from build123d import *

# Parameters (mm, degrees)
F0_R     = 2.54
F1_DEPTH = 2.54
F2_R     = 10.16
F3_DEPTH = 1.27


# Not quite as in the source:
# - a feature names something its author has since deleted; it is built from what else it names


with BuildPart() as f1:
    # F0 (on Front) → F1 (new body)
    with BuildSketch(Plane.XZ):
        with BuildLine():
            ThreePointArc((23.9710795428, 0.5081666473), (11.7817898671, 6.8022195513), (12.4256249974, 20.5054805165))
            ThreePointArc((12.4256249974, 20.5054805165), (0, 44.5693936748), (-12.4256249974, 20.5054805165))
            ThreePointArc((-12.4256249974, 20.5054805165), (-11.7817898671, 6.8022195513), (-23.9710795428, 0.5081666473))
            ThreePointArc((-23.9710795428, 0.5081666473), (-38.5982271537, -22.2846968374), (-11.5454545455, -21.0136471639))
            ThreePointArc((-11.5454545455, -21.0136471639), (0, -13.6044391026), (11.5454545455, -21.0136471639))
            ThreePointArc((11.5454545455, -21.0136471639), (38.5982271537, -22.2846968374), (23.9710795428, 0.5081666473))
        make_face()
        Circle(F0_R, mode=Mode.SUBTRACT)
    extrude(amount=F1_DEPTH)

    # F2 (on face) → F3 (cut)
    with BuildSketch(Plane(origin=(0, 0, 0), x_dir=(-1, 0, 0), z_dir=(0, 1, 0))):
        with Locations((25.4, -14.6646968374)):
            Circle(F2_R)
        with Locations((0, 29.3293936748)):
            Circle(F2_R)
        with Locations((-25.4, -14.6646968374)):
            Circle(F2_R)
    extrude(amount=-F3_DEPTH, mode=Mode.SUBTRACT)


solid = f1.part
CAD build for the part. Positions are in the model's coordinates, mm. A direction names the side the tool comes from. Coordinates: 2 decimals unless noted, no trailing zeros. Loops run counter-clockwise (first coordinate to the right, second up) from the corner with the lowest first, then second, coordinate; pieces in that order, holes last. Notation, with made-up numbers: (45.5, 31) - (55.5, 31) arc R19 cw to (55.5, 38) - close; hole circle Ø10 at (-11, -7). An arc over 180 degrees is marked (long way). Write item = value, one per line. Start each with the question number.
Q1. Flat gauge pins, fed straight in: pin 1 Ø6.5 at (x, z) = (0, 0) entering from -Y; pin 2 Ø16.5 at (x, z) = (25.4, -14.66) entering from +Y; pin 3 Ø1 at (y, z) = (-1.5, 10) entering from +X; pin 4 Ø1.5 at (x, y) = (11.5, -1.5) entering from +Z. Where does each tip first touch, or does it go through?
Q2. Cut at C-C, the plane z = -17. List the corners of the cut face in (x, y), then the cut area to 3 significant figures.
Q3. Cut at A-A, the plane x = 0. List the corners of the cut face in (y, z), then the cut area to 3 significant figures.
Q4. Drill centre lines: L1, parallel to X at y = -0.5, z = -18; L2, parallel to Z at x = -25.4, y = -0.6; L3, parallel to X at y = -1.15, z = -12.5. Where is each one in solid material? Low to high.
Q5. Cut at B-B, the plane x = 25.4. List the corners of the cut face in (y, z).
Q6. Cut at D-D, the plane y = -1.7. List the corners of the cut face in (x, z).
Q7. Which spindle directions (+Z, -Z, +X, -X, +Y, -Y) get a long thin tool onto all of the face, cutting with end or side? Do faces 4 (the cylindrical face through (-38.825, -1.252, -21.877)), 5 (the cylindrical face through (33.5, -0.6, -20.8)). Say none if no direction does.
Q8. Pull direction X, two halves, no side cores. Call faces 1 (the cylindrical face through (0.467, -1.252, 44.562)), 2 (the cylindrical face through (2.2, -0.63, 19.41)), 3 (the flat face through (-1, -2.54, 8)): pulls with the +X half, pulls with the -X half, needs draft (parallel to the pull), parting line crosses it, or undercut.
Computed:
q1.pin_1 = -2.54
q1.pin_2 = -1.27
q1.pin_3 = 10.62
q1.pin_4 = 40.13
q2.outline = (-40.46, -2.54) - (-8.64, -2.54) - (-8.64, 0) - (-15.51, 0) - (-15.51, -1.27) - (-35.29, -1.27) - (-35.29, 0) - (-40.46, 0) - close; (8.64, -2.54) - (40.46, -2.54) - (40.46, 0) - (35.29, 0) - (35.29, -1.27) - (15.51, -1.27) - (15.51, 0) - (8.64, 0) - close
q2.area = 111 mm²
q3.outline = (-2.54, -13.6) - (0, -13.6) - (0, -2.54) - (-2.54, -2.54) - close; (-2.54, 2.54) - (0, 2.54) - (0, 19.17) - (-1.27, 19.17) - (-1.27, 39.49) - (0, 39.49) - (0, 44.57) - (-2.54, 44.57) - close
q3.area = 109 mm²
q4.L1 = -40.27 to -35, -15.8 to -9.61, 9.61 to 15.8, 35 to 40.27
q4.L2 = -29.9 to -24.82, -4.5 to 0.58
q4.L3 = -40.49 to -35.33, -15.47 to 15.47, 35.33 to 40.49
q5.outline = (-2.54, -29.9) - (0, -29.9) - (0, -24.82) - (-1.27, -24.82) - (-1.27, -4.5) - (0, -4.5) - (0, 0.58) - (-2.54, 0.58) - close
q6.outline = (-23.97, 0.51) arc R15.24 ccw (long way) to (-11.55, -21.01) arc R12.7 cw to (11.55, -21.01) arc R15.24 ccw (long way) to (23.97, 0.51) arc R12.7 cw to (12.43, 20.51) arc R15.24 ccw (long way) to (-12.43, 20.51) arc R12.7 cw to start; hole circle Ø5.08 at (0, 0)
q7.face_4 = +Y, -Y
q7.face_5 = +Y
q8.face_1 = parting line crosses it
q8.face_2 = undercut
q8.face_3 = needs draft
